Verification items for this drawing (mm, ordinates from the low corner). A direction names the side the tool comes from. Give positions to 0.01 mm unless a question says otherwise; leave off trailing zeros. Loops run counter-clockwise (first coordinate to the right, second up) from the corner with the lowest first, then second, coordinate; pieces in that order, holes last. Notation, with made-up numbers: (18.5, 5) -> (34.5, 5) arc R23 cw to (34.5, 33) -> close; hole circle Ø9 at (74, -19.75). An arc over 180 degrees is marked (long way). Write each question's results on one line, items separated by ' | '. Start each with the question number.
Item 1: Cross-section at D-D on z = 4. Enter the section's corners in (x, y).
Item 2: Cross-section at C-C on y = 4.25. Enter the section's corners in (x, z).
Item 3: Access from +Z, -Z, +X, -X, +Y, -Y to the whole of each face (thin tool, end or side, straight path). Record for the marked faces 5 and 6.
Item 4: Gauge pin test, flat ends, axial feed: pin 1 Ø1 at (y, z) = (5, 3) entering from -X; pin 2 Ø3 at (x, y) = (9, 3.5) entering from -Z; pin 3 Ø1 at (x, y) = (4.5, 3.5) entering from +Z; pin 4 Ø2 at (y, z) = (5, 8) entering from +X. Record the tip position at first contact, or that the pin passes through.
Item 5: Cross-section at B-B on x = 7.5. Enter the section's corners in (y, z).
Item 6: Scan lines: line 1 along Z through (x, y) = (9.5, 3.75); line 2 along X through (y, z) = (5.25, 6.75); line 3 along Y through (x, z) = (17, 4.5). Record each from-to range of solid material in increasing order.
Item 7: Cross-section at A-A on z = 11.25. Enter the section's corners in (x, y).
Item 8: Mould release check, pull along X, two halves, no side actions. Record for the marked faces 1, 2, 3 and 4: pulls with the +X half, pulls with the -X half, needs draft (parallel to the pull), parting line crosses it, or undercut.
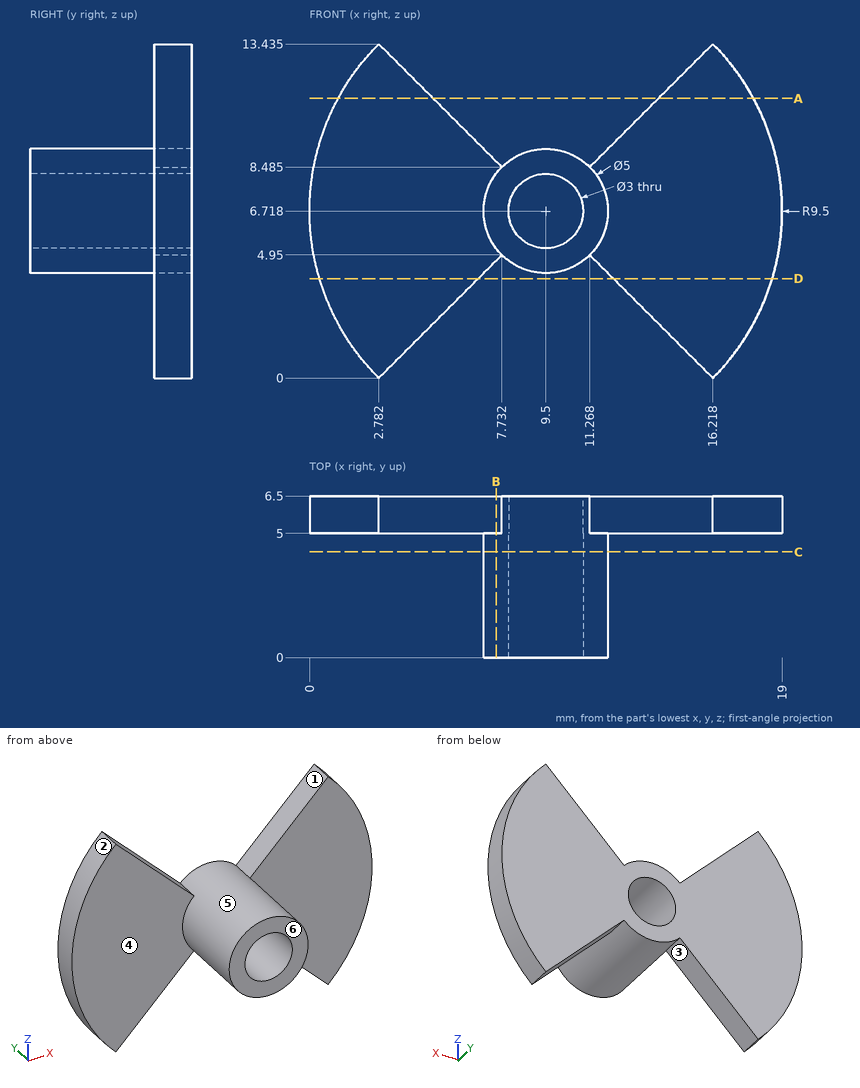
Answer sheet:
1) outline: (0.4, 5) -> (6.78, 5) -> (6.78, 6.5) -> (0.4, 6.5) -> close; (12.22, 5) -> (18.6, 5) -> (18.6, 6.5) -> (12.22, 6.5) -> close
2) outline: circle Ø5 at (9.5, 6.72); hole circle Ø3 at (9.5, 6.72)
3) face 5: -Y | face 6: +Z, -Z, +X, -X, -Y
4) pin 1: stops at x = 0.56 | pin 2: stops at z = 4.22 | pin 3: passes through | pin 4: stops at x = 19
5) outline: (0, 5.22) -> (5, 5.22) -> (5, 4.72) -> (6.5, 4.72) -> (6.5, 8.72) -> (5, 8.72) -> (5, 8.22) -> (0, 8.22) -> close
6) line 1: z = 4.22 to 5.22, 8.22 to 9.22 | line 2: x = 0 to 8, 11 to 19 | line 3: y = 5 to 6.5
7) outline: (1.15, 5) -> (4.97, 5) -> (4.97, 6.5) -> (1.15, 6.5) -> close; (14.03, 5) -> (17.85, 5) -> (17.85, 6.5) -> (14.03, 6.5) -> close
8) face 1: undercut | face 2: pulls with the -X half | face 3: undercut | face 4: needs draft
